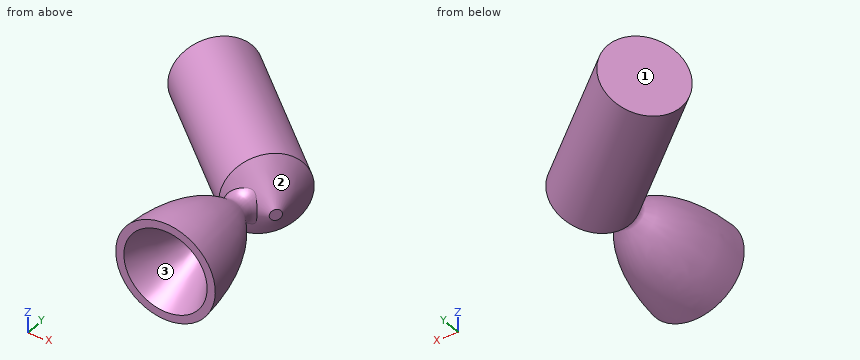
```python
from build123d import *


with BuildPart() as part:
    # Sketch2 → Revolve1 (revolve)
    with BuildSketch(Plane.XY):
        Polygon((1030.061278696, -216.58443678), (959.657201148, -155.39542863), (972.314875011, -140.831508096), (1031.82096691, -192.548949314), (1031.82096691, -214.559739384), align=None)
    revolve(axis=Axis((1030.061278696, -216.58443678, 0), (-0.754774987, 0.655983779, 0)))

    # Sketch1 → Revolve2 (revolve)
    with BuildSketch(Plane.XY, mode=Mode.PRIVATE) as revolve2_sk:
        with BuildLine():
            Line((1034.963586572, -271.3945274), (1038.828918992, -271.3945274))
            add(Edge.make_bspline(
                [(1038.828918992, -271.3945274), (1037.873448174, -256.436961098), (1033.932423541, -239.028318184), (1022.04554778, -226.197270809), (1021.385558194, -223.249921116), (1023.46164644, -215.880421657), (1031.802541842, -213.509952537), (1030.500568899, -206.266042019)],
                knots=[0, 0, 0, 0, 0.648973555, 0.689713178, 0.725948802, 0.770741807, 1, 1, 1, 1], degree=3))
            Line((1030.500568899, -206.266042019), (1015.25039123, -206.266042019))
            Line((1015.25039123, -206.266042019), (1015.25039123, -232.741203199))
            Line((1015.25039123, -232.741203199), (1034.963586572, -271.3945274))
        make_face()
    revolve(revolve2_sk.sketch.rotate(Axis((1015.25039123, -199.885877629, 0), (0, -1, 0)), 270), axis=Axis((1015.25039123, -199.885877629, 0), (0, -1, 0)))  # turned: the seam where the file's is


solid = part.part
```
Here's how the part is built. I have some questions about the finished solid (model axes, mm). Face numbers are marked on the shaded views. Coordinates: 2 decimals unless noted, no trailing zeros. Return JSON: item names as keys, results as strings.
1) I'm going to push flat-ended pins straight in: P1, Ø10, axis at x = 959.5, y = -156.5, coming from the +Z side; P2, Ø2, axis at y = -192, z = 3, coming from the -X side; P3, Ø10, axis at x = 1028.5, z = 12, coming from the +Y side. Where does each tip first touch, or does it pass through?
Conclusion:
{"P1": "stops at z = 19.3", "P2": "stops at x = 971.54", "P3": "stops at y = -189.13"}
2) If I drill on probe 1 along Y at (x, z) = (1012.5, -14); probe 2 along X at (y, z) = (-249, -2.5); probe 3 along Y at (x, z) = (1025, 1.5), over which ranges is the centre line in solid material (lowest first)?
Conclusion:
{"probe 1": "y = -260.72 to -236.19, -216.42 to -183.73", "probe 2": "x = 995.69 to 1007.34, 1023.16 to 1034.81", "probe 3": "y = -252.08 to -229.69, -218.93 to -186.7"}
3) Thinking about a two-plate mould opening in Y: for the marked faces 1, 2 and 3, which applies, +Y half, -Y half, draft (parallel to the pull), parting line (faces both ways), or undercut?
Conclusion:
{"face 1": "+Y half", "face 2": "undercut", "face 3": "-Y half"}
